from build123d import *

# Parameters (mm, degrees)
F1_DEPTH = 340
F2_R     = 10


with BuildPart() as f1:
    # F0 (on Top) → F1 (new body, symmetric)
    with BuildSketch(Plane.XY):
        with BuildLine():
            Line((225, -50), (225, 0))
            ThreePointArc((225, 0), (0, 25.641237), (-225, 0))
            Line((-225, 0), (-225, -50))
            Line((-225, -50), (-156.175058, -266.073386))
            Line((-156.175058, -266.073386), (-50, -314.358763))
            Line((-50, -314.358763), (50, -314.358763))
            Line((50, -314.358763), (171.62508, -204.769474))
            Line((171.62508, -204.769474), (225, -50))
        make_face()
    extrude(amount=F1_DEPTH, both=True)

    # F2
    f2_edges = [f1.edges().sort_by_distance(p)[0] for p in [
        (225, 0, 0),
        (0, 25.641237, -340),
        (-225, 0, 0),
        (0, 25.641237, 340),
        (-225, -25, -340),
        (-225, -50, 0),
        (-225, -25, 340),
        (-190.587529, -158.036693, -340),
        (-156.175058, -266.073386, 0),
        (-190.587529, -158.036693, 340),
        (225, -50, 0),
        (225, -25, -340),
        (225, -25, 340),
        (171.62508, -204.769474, 0),
        (198.31254, -127.384737, -340),
        (198.31254, -127.384737, 340),
        (110.81254, -259.564119, -340),
        (110.81254, -259.564119, 340),
        (50, -314.358763, 0),
        (0, -314.358763, -340),
        (0, -314.358763, 340),
        (-50, -314.358763, 0),
        (-103.087529, -290.216075, -340),
        (-103.087529, -290.216075, 340),
    ]]
    fillet(f2_edges, radius=F2_R)


solid = f1.part
Can you work these out from the model? Positions are in its coordinate system, mm. Round coordinates to 2 decimals unless told otherwise and drop trailing zeros. Order: outer loops, then holes, each group sorted by start corner. A loop starts at its lowest first (then second) coordinate and runs counter-clockwise, first axis right, second up. Notation, with made-up numbers: M -38,12 L -27,12 A33 cw -27,40 Z; hole C -4,86 d8. An arc over 180 degrees is marked long. Use a Markdown table: item, result.
1) If I drill on line 1 along Y through (x, z) = (-33.5, -101.5); line 2 along Y through (x, z) = (117, -81.5); line 3 along X through (y, z) = (-150.5, -209), over which ranges is the centre line in solid material (lowest first)?
Geometry says:
| item | result |
|---|---|
| line 1 | y = -314.36 to 25.08 |
| line 2 | y = -253.99 to 18.77 |
| line 3 | x = -192.99 to 190.34 |
2) I'm going to push flat-ended pins straight in: P1, Ø1.5, axis at y = -275.5, z = -106, coming from the -X side; P2, Ø12, axis at y = -156.5, z = -21, coming from the +X side; P3, Ø4, axis at x = 132, z = -173.5, coming from the +Y side. Where does each tip first touch, or does it pass through?
Geometry says:
| item | result |
|---|---|
| P1 | stops at x = -137.1 |
| P2 | stops at x = 190.34 |
| P3 | stops at y = 17.16 |
3) Imagine slicing it at A-A (z = 12). List the corners of the cut face in (x, y) for me, then the cut area to 3 significant figures.
Geometry says:
| item | result |
|---|---|
| outline | M -225,-48.45 A10 ccw -224.53,-51.48 L -157.52,-261.84 A10 ccw -152.13,-267.91 L -51.97,-313.46 A10 ccw -47.83,-314.36 L 46.16,-314.36 A10 ccw 52.85,-311.79 L 169.71,-206.5 A10 ccw 172.47,-202.33 L 224.45,-51.58 A10 ccw 225,-48.32 L 225,-7.99 A10 ccw 217.17,1.77 A1000 ccw -217.17,1.77 A10 ccw -225,-7.99 Z |
| area | 119,000 mm² |
